The model under review builds one solid part; all positions refer to its coordinate system, in mm. Give positions to 0.01 mm unless a question says otherwise; leave off trailing zeros. Answer as CSV lines item,"result". Start each with the question number.
Autodesk Inventor part; units mm, degrees
ref_plane "Start Plane" through (0, 0, -10) normal (0, 0, 1) x (1, 0, 0)
ref_plane "End Plane" through (0, 0, 510) normal (0, 0, 1) x (1, 0, 0)
ref_plane "Work Plane6" through (-139.969, 0, -10) normal (0, 0, -1) x (-1, 0, 0)
ref_plane "Start Plane" through (0, 0, -10) normal (0, 0, 1) x (1, 0, 0)
ref_plane "End Plane" through (0, 0, 510) normal (0, 0, 1) x (1, 0, 0)
sketch "Sketch" plane through (0, 0, 0) normal (0, 0, 1) x (1, 0, 0)
  line L0 (0, 0) -> (2.5, 0) construction
  line L1 (0, 0) -> (0, 2.5) construction
  line L2 (0, 4) -> (0, -4) construction
  line L3 (0, 4) -> (1.7574, 4)
  arc A0 (1.7574, 4) -> (3.1716, 4.5858) centre (1.7574, 6) ccw
  line L4 (3.1716, 4.5858) -> (5.7322, 7.1464)
  line L5 (-4, 0) -> (4, 0) construction
  line L6 (4, 0) -> (4, 1.7574)
  arc A1 (4.5858, 3.1716) -> (4, 1.7574) centre (6, 1.7574) ccw
  line L7 (4.5858, 3.1716) -> (7.1464, 5.7322)
  line L8 (0, 0) -> (10, 10) construction
  line L9 (0, 0) -> (19.6827, 0) construction
  arc A2 (8, 5.3787) -> (7.1464, 5.7322) centre (7.5, 5.3787) ccw
  line L10 (8, 5.3787) -> (8, 3.5)
  arc A3 (8, 3.5) -> (8.5, 3) centre (8.5, 3.5) ccw
  line L11 (8.5, 3) -> (9.5, 3)
  arc A4 (9.5, 3) -> (10, 3.5) centre (9.5, 3.5) ccw
  line L12 (10, 3.5) -> (10, 9)
  line L13 (10, 9) -> (10, 10) construction
  arc A5 (5.7322, 7.1464) -> (5.3787, 8) centre (5.3787, 7.5) ccw
  line L14 (5.3787, 8) -> (3.5, 8)
  arc A6 (3, 8.5) -> (3.5, 8) centre (3.5, 8.5) ccw
  line L15 (3, 8.5) -> (3, 9.5)
  arc A7 (3.5, 10) -> (3, 9.5) centre (3.5, 9.5) ccw
  line L16 (3.5, 10) -> (9, 10)
  arc A8 (10, 9) -> (9, 10) centre (9, 9) ccw
  line L17 (0, 4) -> (-1.7574, 4)
  arc A9 (-3.1716, 4.5858) -> (-1.7574, 4) centre (-1.7574, 6) ccw
  line L18 (-3.1716, 4.5858) -> (-5.7322, 7.1464)
  line L19 (-4, 0) -> (-4, 1.7574)
  arc A10 (-4, 1.7574) -> (-4.5858, 3.1716) centre (-6, 1.7574) ccw
  line L20 (-4.5858, 3.1716) -> (-7.1464, 5.7322)
  arc A11 (-7.1464, 5.7322) -> (-8, 5.3787) centre (-7.5, 5.3787) ccw
  line L21 (-8, 5.3787) -> (-8, 3.5)
  arc A12 (-8.5, 3) -> (-8, 3.5) centre (-8.5, 3.5) ccw
  line L22 (-8.5, 3) -> (-9.5, 3)
  arc A13 (-10, 3.5) -> (-9.5, 3) centre (-9.5, 3.5) ccw
  line L23 (-10, 3.5) -> (-10, 9)
  arc A14 (-5.3787, 8) -> (-5.7322, 7.1464) centre (-5.3787, 7.5) ccw
  line L24 (-5.3787, 8) -> (-3.5, 8)
  arc A15 (-3.5, 8) -> (-3, 8.5) centre (-3.5, 8.5) ccw
  line L25 (-3, 8.5) -> (-3, 9.5)
  arc A16 (-3, 9.5) -> (-3.5, 10) centre (-3.5, 9.5) ccw
  line L26 (-3.5, 10) -> (-9, 10)
  arc A17 (-9, 10) -> (-10, 9) centre (-9, 9) ccw
  line L27 (0, -4) -> (-1.7574, -4)
  arc A18 (-1.7574, -4) -> (-3.1716, -4.5858) centre (-1.7574, -6) ccw
  line L28 (-3.1716, -4.5858) -> (-5.7322, -7.1464)
  arc A19 (-5.7322, -7.1464) -> (-5.3787, -8) centre (-5.3787, -7.5) ccw
  line L29 (-5.3787, -8) -> (-3.5, -8)
  arc A20 (-3, -8.5) -> (-3.5, -8) centre (-3.5, -8.5) ccw
  line L30 (-3, -8.5) -> (-3, -9.5)
  arc A21 (-3.5, -10) -> (-3, -9.5) centre (-3.5, -9.5) ccw
  line L31 (-3.5, -10) -> (-9, -10)
  arc A22 (-10, -9) -> (-9, -10) centre (-9, -9) ccw
  line L32 (-10, -3.5) -> (-10, -9)
  arc A23 (-9.5, -3) -> (-10, -3.5) centre (-9.5, -3.5) ccw
  line L33 (-8.5, -3) -> (-9.5, -3)
  arc A24 (-8, -3.5) -> (-8.5, -3) centre (-8.5, -3.5) ccw
  line L34 (-8, -5.3787) -> (-8, -3.5)
  arc A25 (-8, -5.3787) -> (-7.1464, -5.7322) centre (-7.5, -5.3787) ccw
  line L35 (-4.5858, -3.1716) -> (-7.1464, -5.7322)
  arc A26 (-4.5858, -3.1716) -> (-4, -1.7574) centre (-6, -1.7574) ccw
  line L36 (-4, 0) -> (-4, -1.7574)
  line L37 (3.5, -10) -> (9, -10)
  arc A27 (9, -10) -> (10, -9) centre (9, -9) ccw
  line L38 (10, -3.5) -> (10, -9)
  arc A28 (10, -3.5) -> (9.5, -3) centre (9.5, -3.5) ccw
  line L39 (8.5, -3) -> (9.5, -3)
  arc A29 (8.5, -3) -> (8, -3.5) centre (8.5, -3.5) ccw
  line L40 (8, -5.3787) -> (8, -3.5)
  arc A30 (7.1464, -5.7322) -> (8, -5.3787) centre (7.5, -5.3787) ccw
  line L41 (4.5858, -3.1716) -> (7.1464, -5.7322)
  arc A31 (4, -1.7574) -> (4.5858, -3.1716) centre (6, -1.7574) ccw
  line L42 (4, 0) -> (4, -1.7574)
  line L43 (5.3787, -8) -> (3.5, -8)
  arc A32 (5.3787, -8) -> (5.7322, -7.1464) centre (5.3787, -7.5) ccw
  line L44 (3.1716, -4.5858) -> (5.7322, -7.1464)
  arc A33 (3.1716, -4.5858) -> (1.7574, -4) centre (1.7574, -6) ccw
  line L45 (0, -4) -> (1.7574, -4)
  arc A34 (3.5, -8) -> (3, -8.5) centre (3.5, -8.5) ccw
  line L46 (3, -8.5) -> (3, -9.5)
  arc A35 (3, -9.5) -> (3.5, -10) centre (3.5, -9.5) ccw
  circle A36 centre (0, 0) radius 2.5
  dimension "d1" = 8
  dimension "d2" = 2
  dimension "d3" = 8
  dimension "d4" = 2
  dimension "d5" = 2
  dimension "d7" = 45
  dimension "d8" = 0.5
  dimension "d9" = 0.5
  dimension "d10" = 0.5
  dimension "d12" = 2
  dimension "d17" = 7
  dimension "d18" = 10
  dimension "d19" = 0.5
  dimension "d20" = 1
  dimension "d21" = 0.5
  dimension "d22" = 0.5
  dimension "d23" = 2
  dimension "d24" = 7
  dimension "d25" = 5
extrude "Body" add sketch "Sketch" along normal up to surface (520 mm away) from surface at -10
sketch "Sketch6" plane through (0, 0, 0) normal (0, 0, 1) x (1, 0, 0)
  line L0 (0, 0) -> (10, 0)
ref_plane "Work Plane5" through (0, 0, 0) normal (0, -1, 0) x (1, 0, 0)
sketch "Sketch7" plane through (0, 0, 0) normal (0, -1, 0) x (1, 0, 0)
  line L0 (-2, -10) -> (12, -10)
  line L1 (-2, 510) -> (12, 510)
  dimension "d33" = 520
ref_plane "Work Plane6" through (-139.969, 0, -10) normal (0, 0, -1) x (-1, 0, 0)
split "Split1" plane through (-139.969, 0, -10) removes the side toward (0, 0, -1)
ref_plane "Work Plane7" through (-10.031, 0, 510) normal (0, 0, 1) x (1, 0, 0)
split "Split2" plane through (-10.031, 0, 510) removes the side toward (0, 0, 1)
equation "\"d1\" = 0.8 * sigma"
equation "\"d2\" = 0.2 * sigma"
equation "\"d3\" = 0.8 * sigma"
equation "\"d4\" = 0.2 * sigma"
equation "\"d5\" = 0.2 * sigma"
equation "\"d8\" = 0.05 * sigma"
equation "\"d9\" = 0.05 * sigma"
equation "\"d10\" = 0.05 * sigma"
equation "\"d12\" = 0.2 * sigma"
equation "\"d17\" = 0.7 * sigma"
equation "\"d18\" = sigma"
equation "\"d19\" = 0.05 * sigma"
equation "\"d20\" = 0.1 * sigma"
equation "\"d21\" = 0.05 * sigma"
equation "\"d22\" = 0.05 * sigma"
equation "\"d23\" = 0.2 * sigma"
equation "\"d24\" = 0.7 * sigma"
equation "\"d25\" = 0.5 * sigma"
equation "\"sigma\" = 1"
equation "\"G_L\" = d33"
properties part number "A3.3-MEM"
Item 1: Clearance check with flat-ended pins moving along their axes: pin 1 (1.8 mm diameter, centred on x = 0.5, z = 136.5, fed in from -Y); pin 2 (1.1 mm diameter, centred on y = 0.5, z = 309, fed in from +X). State where each tip first meets the part, or that it passes through.
Item 2: Mouldability with a two-part tool opening along Z and no side actions: class faces 1 (the face through (2, 2, 510)), 2 (the face through (2, 2, -10)) as released by +Z, released by -Z, zero draft, split by the parting line, or undercut.
Item 3: For line 1 along Y through (x, z) = (-4.5, 118); line 2 along Y through (x, z) = (0, 137); line 3 along Y through (x, z) = (-9, 426.5), list the stretches that pass through material, from the lowest coordinate up.
Data:
1,pin 1,"stops at y = -4"
1,pin 2,"stops at x = 4"
2,face 1,"released by +Z"
2,face 2,"released by -Z"
3,line 1,"y = -10 to -8, -5.91 to -3.08, 3.08 to 5.91, 8 to 10"
3,line 2,"y = -4 to -2.5, 2.5 to 4"
3,line 3,"y = -10 to -3, 3 to 10"
